The drawing under review shows one solid part. Ordinate dimensions are in mm from its lowest x, y, z. Give positions to 0.01 mm unless a question says otherwise; leave off trailing zeros. Write each loop counter-clockwise with the first axis right and the second up, starting at its lowest first coordinate (ties: lowest second). Pieces come first, ordered by that corner, then holes. Notation, with made-up numbers: (60.5, 53) - (65.5, 53) arc R21 ccw to (65.5, 69) - close; hole circle Ø4 at (-29.5, 72). An arc over 180 degrees is marked (long way). Write item = value, one per line.
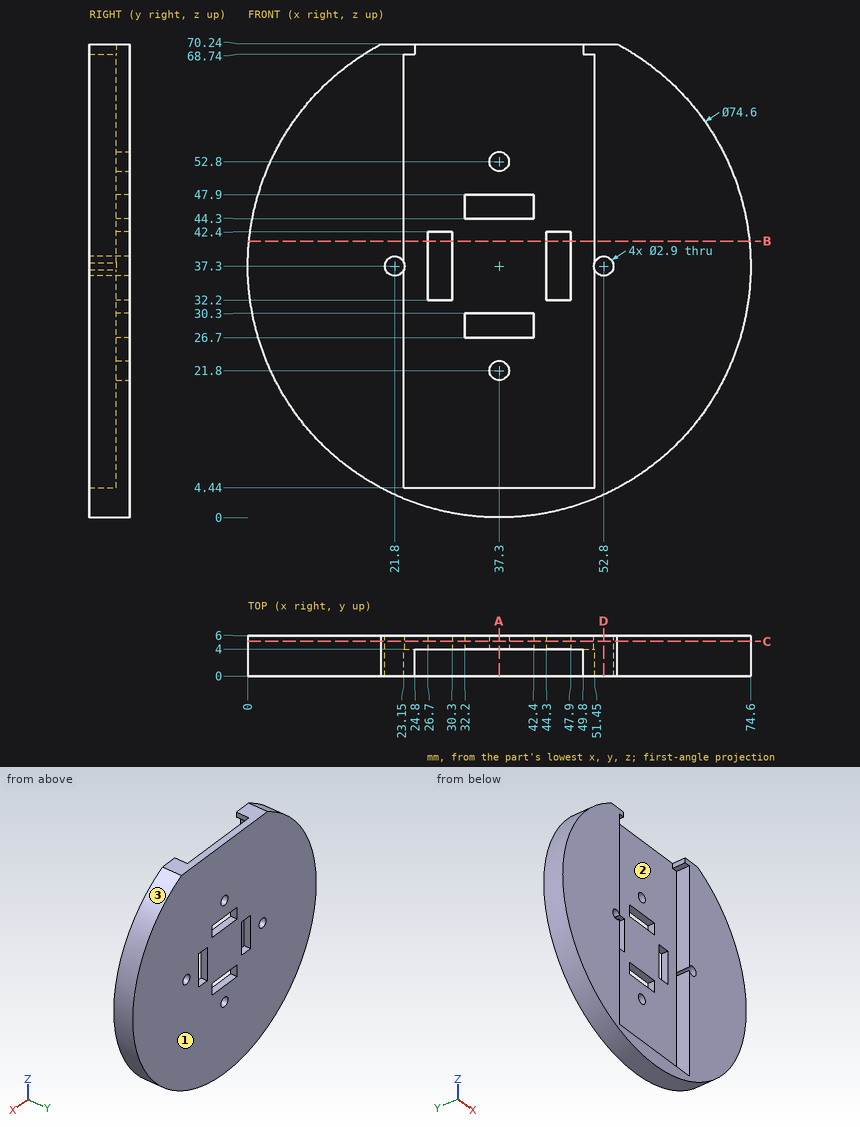
1. Take a section at A-A on x = 37.3. Give the boundary of the cut face in (y, z).
Findings below:
outline = (0, 0) - (6, 0) - (6, 20.35) - (4, 20.35) - (4, 4.44) - (0, 4.44) - close; (4, 23.25) - (6, 23.25) - (6, 26.7) - (4, 26.7) - close; (4, 30.3) - (6, 30.3) - (6, 44.3) - (4, 44.3) - close; (4, 47.9) - (6, 47.9) - (6, 51.35) - (4, 51.35) - close; (4, 54.25) - (6, 54.25) - (6, 70.24) - (4, 70.24) - close
2. Draft analysis for pull direction X (two halves, no side actions). For the marked faces 1, 2 and 3, state which applies: +X half, -X half, draft (parallel to the pull), parting line (faces both ways), or undercut.
Findings below:
face_1 = draft
face_2 = undercut
face_3 = parting line
3. Take a section at C-C on y = 5.15. Count the separate pieces of the cut face and the enclosed holes in it, and give its area (3 significant figures).
Findings below:
separate_pieces = 1
enclosed_holes = 8
area = 4,090 mm²
4. Insertion check: P1, Ø2, axis at y = 5, z = 39.5, coming from the -X side; P2, Ø0.8, axis at y = 1.5, z = 70, coming from the +X side (1 decimal); P3, Ø0.6, axis at y = 5, z = 29, coming from the +X side. Each pin has a flat end and moves straight along its axis. Give the tip position at first contact, or say it passes through.
Findings below:
P1 = 0.02
P2 = 56
P3 = 73.73
5. Take a section at D-D on x = 52.8. Give the boundary of the cut face in (y, z).
Findings below:
outline = (0, 3.37) - (6, 3.37) - (6, 35.85) - (0, 35.85) - close; (0, 38.75) - (6, 38.75) - (6, 70.24) - (0, 70.24) - close
6. For line 1 (Z direction, x = 37.3, y = 4.85); line 2 (X direction, y = 1.4, z = 37.3); line 3 (X direction, y = 5.75, z = 35.5), list the stretches that pass through material, from the lowest coordinate up. Write a range as from..to.
Findings below:
line_1 = 0..20.35, 23.25..26.7, 30.3..44.3, 47.9..51.35, 54.25..70.24
line_2 = 0..20.35, 54.25..74.6
line_3 = 0.04..26.7, 30.3..44.3, 47.9..74.56
7. Take a section at B-B on z = 41. Give the boundary of the cut face in (x, y), and give its area (3 significant figures).
Findings below:
outline = (0.18, 0) - (23.15, 0) - (23.15, 4) - (26.7, 4) - (26.7, 6) - (0.18, 6) - close; (30.3, 4) - (44.3, 4) - (44.3, 6) - (30.3, 6) - close; (47.9, 4) - (51.45, 4) - (51.45, 0) - (74.42, 0) - (74.42, 6) - (47.9, 6) - close
area = 318 mm²
